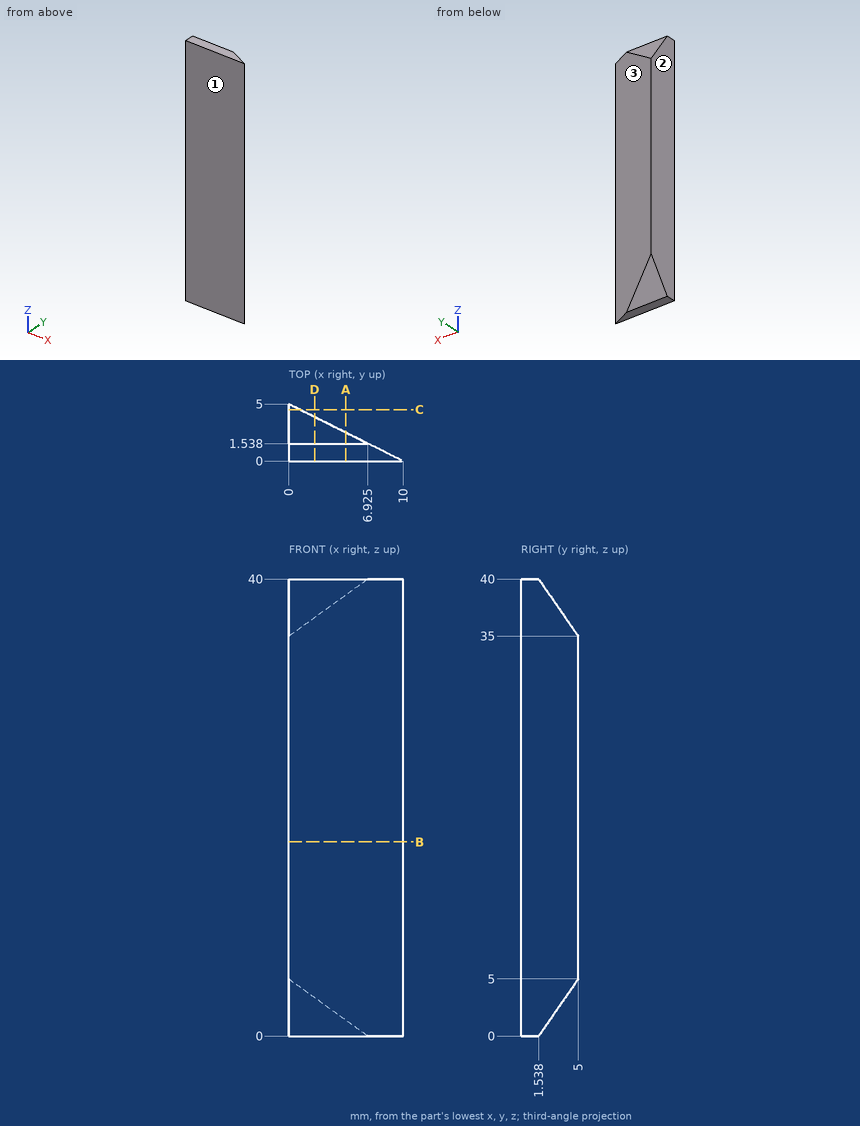
Here's the drawing with two shaded views (mm, measured from the low corner). I have some questions. Give positions to 0.01 mm unless a question says otherwise; leave off trailing zeros. Loops run counter-clockwise (first coordinate to the right, second up) from the corner with the lowest first, then second, coordinate; pieces in that order, holes last. Notation, with made-up numbers: M 47.5,-33 L 88.5,-33 A35 ccw 88.5,-1 Z; hole C 18.25,-31.75 d5. An arc over 180 degrees is marked long. One line per item, written item: value.
1) I'm going to push flat-ended pins straight in: pin 1 (4 mm diameter, centred on x = 3.5, z = 15.5, fed in from +Y); pin 2 (1 mm diameter, centred on x = 8, z = 14, fed in from +Y). Where does each tip first touch, or does it pass through?
Geometry check:
pin 1: stops at y = 4.25
pin 2: stops at y = 1.25
2) Imagine slicing it at A-A on x = 5. Write out the boundary of the cut face in (y, z).
Geometry check:
outline: M 0,0 L 1.54,0 L 2.5,1.39 L 2.5,38.61 L 1.54,40 L 0,40 Z
3) Imagine slicing it at D-D on x = 2.25. Write out the boundary of the cut face in (y, z) (1 decimal).
Geometry check:
outline: M 0,0 L 1.5,0 L 3.9,3.4 L 3.9,36.6 L 1.5,40 L 0,40 Z
4) Thinking about a two-plate mould opening in Y: for the marked faces 1, 2 and 3, which applies, +Y half, -Y half, draft (parallel to the pull), parting line (faces both ways), or undercut?
Geometry check:
face 1: -Y half
face 2: draft
face 3: +Y half
5) Please list where these lines run through material, in increasing order: line 1 (X direction, y = 4.55, z = 14.5); line 2 (Z direction, x = 5.75, y = 2) (1 decimal); line 3 (X direction, y = 4.3, z = 33).
Geometry check:
line 1: x = 0 to 0.9
line 2: z = 0.7 to 39.3
line 3: x = 0 to 1.4
6) Imagine slicing it at B-B on z = 17. Write out the boundary of the cut face in (x, y), and give its area (3 significant figures).
Geometry check:
outline: M 0,0 L 10,0 L 0,5 Z
area: 25.0 mm²
7) Imagine slicing it at C-C on y = 4.5. Write out the boundary of the cut face in (x, z).
Geometry check:
outline: M 0,4.28 L 1,4.28 L 1,35.72 L 0,35.72 Z
